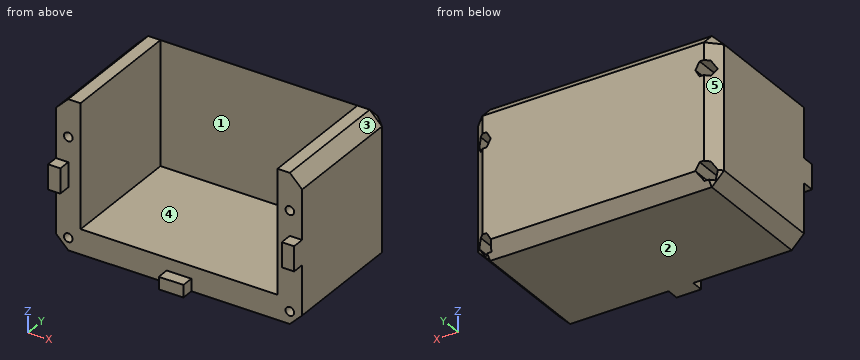
```python
from build123d import *

# Parameters (mm, degrees)
SKETCH1_W               = 100
SKETCH1_H               = 60
BOSS_EXTRUDE1_DEPTH     = 55
CUT_EXTRUDE1_START      = 30
SKETCH2_W               = 80
SKETCH2_H               = 50
CUT_EXTRUDE1_DEPTH      = 50
CHAMFER2_SIZE           = 5
CUT_EXTRUDE2_DEPTH      = 81.156097709
CUT_EXTRUDE2_DEPTH_BACK = 81.156097709
SKETCH3_R               = 1.75
CUT_EXTRUDE3_START      = 55
CUT_EXTRUDE3_DEPTH      = 50
BOSS_EXTRUDE2_START     = -50
SKETCH5_W               = 10
SKETCH5_H               = 5
BOSS_EXTRUDE2_DEPTH     = 5
BOSS_EXTRUDE3_START     = 50
SKETCH5_2_W             = 10
SKETCH5_2_H             = 5
BOSS_EXTRUDE3_DEPTH     = 5
BOSS_EXTRUDE4_START     = -30
SKETCH7_W               = 10
SKETCH7_H               = 5
BOSS_EXTRUDE4_DEPTH     = 5


with BuildPart() as part:
    # Sketch1 → Boss-Extrude1 (new body)
    with BuildSketch(Plane(origin=(0, 0, 0), x_dir=(1, 0, 0), z_dir=(0, 1, 0))):
        Rectangle(SKETCH1_W, SKETCH1_H)
    extrude(amount=BOSS_EXTRUDE1_DEPTH)

    # Sketch2 → Cut-Extrude1 (cut)
    with BuildSketch(Plane.XY.offset(CUT_EXTRUDE1_START)):
        with Locations((0, 25)):
            Rectangle(SKETCH2_W, SKETCH2_H)
    extrude(amount=-CUT_EXTRUDE1_DEPTH, mode=Mode.SUBTRACT)

    # Chamfer2
    chamfer2_edges = [part.edges().sort_by_distance(p)[0] for p in [
        (-50, 55, 0),
        (0, 55, 30),
        (50, 55, 0),
        (50, 27.5, 30),
        (-50, 27.5, 30),
        (-50, 27.5, -30),
        (50, 27.5, -30),
        (0, 55, -30),
    ]]
    chamfer(chamfer2_edges, length=CHAMFER2_SIZE - 0.0001)  # a hair under: the kernel refuses the full size

    # Sketch3 → Cut-Extrude2 (cut, two sides: drawn at the far end of the back side and taken through both)
    with BuildSketch(Plane(origin=(0, 0, 0), x_dir=(1, 0, 0), z_dir=(0, 1, 0)).offset(-CUT_EXTRUDE2_DEPTH_BACK)):
        with Locations(Location((-45, 25, 0), (0, 0, 90))):
            Circle(SKETCH3_R)
        with Locations(Location((45, 25, 0), (0, 0, 90))):
            Circle(SKETCH3_R)
        with Locations(Location((45, -15, 0), (0, 0, 90))):
            Circle(SKETCH3_R)
        with Locations(Location((-45, -15, 0), (0, 0, 90))):
            Circle(SKETCH3_R)
    extrude(amount=CUT_EXTRUDE2_DEPTH + CUT_EXTRUDE2_DEPTH_BACK, mode=Mode.SUBTRACT)

    # Sketch4 → Cut-Extrude3 (cut)
    with BuildSketch(Plane(origin=(0, 0, 0), x_dir=(1, 0, 0), z_dir=(0, 1, 0)).offset(CUT_EXTRUDE3_START)):
        Polygon((-41.535898385, 25), (-43.267949192, 28), (-46.732050808, 28), (-48.464101615, 25), (-46.732050808, 22), (-43.267949192, 22), align=None)
        Polygon((-41.535898385, -15), (-43.267949192, -12), (-46.732050808, -12), (-48.464101615, -15), (-46.732050808, -18), (-43.267949192, -18), align=None)
        Polygon((48.464101615, 25), (46.732050808, 28), (43.267949192, 28), (41.535898385, 25), (43.267949192, 22), (46.732050808, 22), align=None)
        Polygon((48.464101615, -15), (46.732050808, -12), (43.267949192, -12), (41.535898385, -15), (43.267949192, -18), (46.732050808, -18), align=None)
    extrude(amount=-CUT_EXTRUDE3_DEPTH, mode=Mode.SUBTRACT)

    # Sketch5 → Boss-Extrude2 (add)
    with BuildSketch(Plane(origin=(0, 0, 0), x_dir=(0, 0, -1), z_dir=(1, 0, 0)).offset(BOSS_EXTRUDE2_START)):
        with Locations((0, -2.5)):
            Rectangle(SKETCH5_W, SKETCH5_H)
    extrude(amount=BOSS_EXTRUDE2_DEPTH)

    # Sketch5<2> → Boss-Extrude3 (add)
    with BuildSketch(Plane(origin=(0, 0, 0), x_dir=(0, 0, -1), z_dir=(1, 0, 0)).offset(BOSS_EXTRUDE3_START)):
        with Locations((0, -2.5)):
            Rectangle(SKETCH5_2_W, SKETCH5_2_H)
    extrude(amount=-BOSS_EXTRUDE3_DEPTH)

    # Sketch7 → Boss-Extrude4 (add)
    with BuildSketch(Plane.XY.offset(BOSS_EXTRUDE4_START)):
        with Locations((0, -2.5)):
            Rectangle(SKETCH7_W, SKETCH7_H)
    extrude(amount=BOSS_EXTRUDE4_DEPTH)


solid = part.part
```
CAD build for the part. Positions are in the model's coordinates, mm. Face numbers are marked on the shaded views. A direction names the side the tool comes from. Round coordinates to 2 decimals unless told otherwise and drop trailing zeros. One line per question, with ' | ' between items.
Q1. Which spindle directions (+Z, -Z, +X, -X, +Y, -Y) get a long thin tool onto all of the face, cutting with end or side? Do the marked faces 1 and 2. Say none if no direction does.
Completed:
face 1: +Z, -Y | face 2: -Z, +X, -X, +Y, -Y
Q2. Slice it at B-B (y = 26). Give the number of separate pieces and of enclosed holes in the cut face, then the cut area to 3 significant figures.
Completed:
separate pieces: 1 | enclosed holes: 4 | area: 1,830 mm^2
Q3. Drop flat-ended pins along their axis: pin 1 (12 mm diameter, centred on x = 0, z = -7.5, fed in from -Y); pin 2 (5 mm diameter, centred on x = -46, z = 15, fed in from +Y); pin 3 (4 mm diameter, centred on x = 46.5, y = -2.5, fed in from +Z); pin 4 (6.5 mm diameter, centred on x = 45, z = 15, fed in from +Y). Give the stop position or say it passes through.
Completed:
pin 1: stops at y = 50 | pin 2: stops at y = 52.8 | pin 3: stops at z = 5 | pin 4: stops at y = 55
Q4. Probe probe 1 along X at (y, z) = (3.6, -25); probe 2 along X at (y, z) = (3, 15); probe 3 along X at (y, z) = (34, -3.5). List the from-to ranges inside material, lowest first.
Completed:
probe 1: x = -50 to -46.75, -43.25 to 43.25, 46.75 to 50 | probe 2: x = -50 to -46.75, -43.25 to -40, 40 to 43.25, 46.75 to 50 | probe 3: x = -50 to -40, 40 to 50
Q5. Two-plate mould, pull along X, no slides. Class the marked faces 3, 4 and 5: released by +X, released by -X, zero draft, split by the parting line, or undercut.
Completed:
face 3: released by +X | face 4: undercut | face 5: released by -X
